from build123d import *

# Parameters (mm, degrees)
SKETCH_1_W                = 50
SKETCH_1_H                = 80
EXTRUDE_1_DEPTH           = 20
CUT_EXTRUDE_1_DEPTH       = 18
CUT_EXTRUDE_1_DEPTH_BACK  = 48
SKETCH_2_W                = 40
SKETCH_2_H                = 40
CUT_EXTRUDE_2_DEPTH       = 25
CUT_EXTRUDE_2_DEPTH_BACK  = 50
SKETCH_3_R                = 1.45
SKETCH_5_W                = 20
SKETCH_5_H                = 20
EXTRUDE_3_DEPTH           = 10
SKETCH_6_W                = 20
SKETCH_6_H                = 20
EXTRUDE_4_DEPTH           = 10
SKETCH_11_W               = 70
SKETCH_11_H               = 5
EXTRUDE_6_DEPTH           = 20
SKETCH_12_R               = 2.5
CUT_EXTRUDE_6_DEPTH       = 26
CHAMFER_1_SIZE            = 10
SKETCH_14_W               = 25
SKETCH_14_H               = 15
EXTRUDE_7_DEPTH           = 20
CHAMFER_2_SIZE            = 3
CHAMFER_3_SIZE            = 2
CUT_EXTRUDE_8_DEPTH       = 30
CUT_EXTRUDE_8_DEPTH_BACK  = 57
SKETCH_17_R               = 1.45
SKETCH_18_W               = 26.067158979
SKETCH_18_H               = 13.506639349
CUT_EXTRUDE_9_DEPTH       = 42
SKETCH_19_RX              = 28.99919082
SKETCH_19_RY              = 15.360713199
CUT_EXTRUDE_10_DEPTH      = 42
FILLET_1_R                = 7
EXTRUDE_START             = -12
SKETCH_20_R               = 2.5
SKETCH_20_R_2             = 1.75
EXTRUDE_8_DEPTH           = 3.5
SKETCH_21_W               = 20
SKETCH_21_H               = 0.5
CUT_EXTRUDE_11_DEPTH      = 31
SKETCH_22_W               = 50
SKETCH_22_H               = 2
CUT_EXTRUDE_12_DEPTH      = 31
CUT_EXTRUDE_14_DEPTH      = 14
CUT_EXTRUDE_14_DEPTH_BACK = 53
SKETCH_24_R               = 1.45
SKETCH_25_R               = 1.45
CUT_EXTRUDE_16_DEPTH      = 26
SKETCH_26_R               = 4
CUT_EXTRUDE_17_DEPTH      = 10


with BuildPart() as part:
    # 草图1 → 凸台-拉伸1 (new body)
    with BuildSketch(Plane.XY):
        Rectangle(SKETCH_1_W, SKETCH_1_H)
    extrude(amount=EXTRUDE_1_DEPTH)

    # 草图2 → 切除-拉伸1 (cut, two sides: drawn at the far end of the back side and taken through both)
    with BuildSketch(Plane.XY.offset(20).offset(-CUT_EXTRUDE_1_DEPTH_BACK)):
        with Locations((-25, 0)):
            Rectangle(SKETCH_2_W, SKETCH_2_H)
        with Locations((25, 0)):
            Rectangle(SKETCH_2_W, SKETCH_2_H)
    extrude(amount=CUT_EXTRUDE_1_DEPTH + CUT_EXTRUDE_1_DEPTH_BACK, mode=Mode.SUBTRACT)

    # 草图3 → 切除-拉伸2 (cut, two sides: drawn at the far end of the back side and taken through both)
    with BuildSketch(Plane.XY.offset(20).offset(-CUT_EXTRUDE_2_DEPTH_BACK)):
        with Locations(Location((9.925, -24.661145618, 0), (0, 0, 180))):
            Circle(SKETCH_3_R)
        with Locations(Location((19.775, -24.661145618, 0), (0, 0, 180))):
            Circle(SKETCH_3_R)
        with Locations(Location((9.925, 24.761145618, 0), (0, 0, 180))):
            Circle(SKETCH_3_R)
        with Locations(Location((19.775, 24.761145618, 0), (0, 0, 180))):
            Circle(SKETCH_3_R)
        with Locations(Location((-9.925, 24.761145618, 0), (0, 0, 180))):
            Circle(SKETCH_3_R)
        with Locations(Location((-19.775, 24.761145618, 0), (0, 0, 180))):
            Circle(SKETCH_3_R)
        with Locations(Location((-9.925, -24.661145618, 0), (0, 0, 180))):
            Circle(SKETCH_3_R)
        with Locations(Location((-19.775, -24.661145618, 0), (0, 0, 180))):
            Circle(SKETCH_3_R)
    extrude(amount=CUT_EXTRUDE_2_DEPTH + CUT_EXTRUDE_2_DEPTH_BACK, mode=Mode.SUBTRACT)

    # 草图5 → 凸台-拉伸3 (add)
    with BuildSketch(Plane(origin=(25, 0, 0), x_dir=(0, 0, -1), z_dir=(1, 0, 0))):
        with Locations((-10, -30)):
            Rectangle(SKETCH_5_W, SKETCH_5_H)
    extrude(amount=EXTRUDE_3_DEPTH)

    # 草图6 → 凸台-拉伸4 (add)
    with BuildSketch(Plane.ZY.offset(25)):
        with Locations((10, -30)):
            Rectangle(SKETCH_6_W, SKETCH_6_H)
    extrude(amount=EXTRUDE_4_DEPTH)

    # 草图11 → 凸台-拉伸6 (add)
    with BuildSketch(Plane.XY.offset(20)):
        with Locations((0, -42.5)):
            Rectangle(SKETCH_11_W, SKETCH_11_H)
    extrude(amount=-EXTRUDE_6_DEPTH)

    # 草图12 → 切除-拉伸6 (cut)
    with BuildSketch(Plane.XY.offset(20)):
        with Locations((27, -37)):
            Circle(SKETCH_12_R)
        with Locations(Location((-27, -37, 0), (0, 0, 180))):
            Circle(SKETCH_12_R)
    extrude(amount=-CUT_EXTRUDE_6_DEPTH, mode=Mode.SUBTRACT)

    # 倒角1
    chamfer_1_edges = [part.edges().sort_by_distance(p)[0] for p in [
        (35, -20, 10),
        (-35, -20, 10),
    ]]
    chamfer(chamfer_1_edges, length=CHAMFER_1_SIZE)

    # 草图14 → 凸台-拉伸7 (add)
    with BuildSketch(Plane.XY.offset(20)):
        with Locations((0, -45)):
            Rectangle(SKETCH_14_W, SKETCH_14_H)
    extrude(amount=-EXTRUDE_7_DEPTH)

    # 倒角2
    chamfer_2_edges = [part.edges().sort_by_distance(p)[0] for p in [
        (12.5, -52.5, 10),
        (-12.5, -52.5, 10),
    ]]
    chamfer(chamfer_2_edges, length=CHAMFER_2_SIZE)

    # 倒角3
    chamfer_3_edges = [part.edges().sort_by_distance(p)[0] for p in [
        (0, -52.5, 0),
        (0, -52.5, 20),
    ]]
    chamfer(chamfer_3_edges, length=CHAMFER_3_SIZE)

    # 草图17 → 切除-拉伸8 (cut, two sides: drawn at the far end of the back side and taken through both)
    with BuildSketch(Plane(origin=(0, 0, 0), x_dir=(-1, 0, 0), z_dir=(0, 0, -1)).offset(-CUT_EXTRUDE_8_DEPTH_BACK)):
        with Locations((15, 33)):
            Circle(SKETCH_17_R)
        with Locations((-15, 33)):
            Circle(SKETCH_17_R)
    extrude(amount=CUT_EXTRUDE_8_DEPTH + CUT_EXTRUDE_8_DEPTH_BACK, mode=Mode.SUBTRACT)

    # 草图18 → 切除-拉伸9 (cut)
    with BuildSketch(Plane.XY.offset(20)):
        with Locations((-0.53357949, -51.753319675)):
            Rectangle(SKETCH_18_W, SKETCH_18_H)
    extrude(amount=-CUT_EXTRUDE_9_DEPTH, mode=Mode.SUBTRACT)

    # 草图19 → 切除-拉伸10 (cut)
    with BuildSketch(Plane.XY.offset(20)):
        with Locations(Location((0, -56.905793797), (0, 0, 0))):
            Ellipse(SKETCH_19_RX, SKETCH_19_RY)
    extrude(amount=-CUT_EXTRUDE_10_DEPTH, mode=Mode.SUBTRACT)

    # 圆角1
    fillet_1_edges = [part.edges().sort_by_distance(p)[0] for p in [
        (-35, -45, 10),
        (35, -45, 10),
    ]]
    fillet(fillet_1_edges, radius=FILLET_1_R)

    # 草图20 → 凸台-拉伸8 (add)
    # profile 1 of 2: a face of its own
    with BuildSketch(Plane(origin=(0, 0, 0), x_dir=(-1, 0, 0), z_dir=(0, 0, -1)).offset(EXTRUDE_START)):
        with Locations((27, -37)):
            Circle(SKETCH_20_R)
        with Locations((27, -37)):
            Circle(SKETCH_20_R_2, mode=Mode.SUBTRACT)
    # profile 2 of 2: a face of its own
    with BuildSketch(Plane(origin=(0, 0, 0), x_dir=(-1, 0, 0), z_dir=(0, 0, -1)).offset(EXTRUDE_START)):
        with Locations(Location((-27, -37, 0), (0, 0, 180))):
            Circle(SKETCH_20_R)
        with Locations((-27, -37)):
            Circle(SKETCH_20_R_2, mode=Mode.SUBTRACT)
    extrude(amount=EXTRUDE_8_DEPTH)

    # 草图21 → 切除-拉伸11 (cut)
    with BuildSketch(Plane(origin=(0, 0, 0), x_dir=(-1, 0, 0), z_dir=(0, 0, -1))):
        with Locations((-15, 20.25)):
            Rectangle(SKETCH_21_W, SKETCH_21_H)
        with Locations((15, 20.25)):
            Rectangle(SKETCH_21_W, SKETCH_21_H)
    extrude(amount=-CUT_EXTRUDE_11_DEPTH, mode=Mode.SUBTRACT)

    # 草图22 → 切除-拉伸12 (cut)
    with BuildSketch(Plane(origin=(0, 0, 0), x_dir=(-1, 0, 0), z_dir=(0, 0, -1))):
        with Locations((0, 39)):
            Rectangle(SKETCH_22_W, SKETCH_22_H)
    extrude(amount=-CUT_EXTRUDE_12_DEPTH, mode=Mode.SUBTRACT)

    # 草图24 → 切除-拉伸14 (cut, two sides: drawn at the far end of the back side and taken through both)
    with BuildSketch(Plane(origin=(0, 0, 0), x_dir=(-1, 0, 0), z_dir=(0, 0, -1)).offset(-CUT_EXTRUDE_14_DEPTH_BACK)):
        with Locations((0, -33)):
            Circle(SKETCH_24_R)
    extrude(amount=CUT_EXTRUDE_14_DEPTH + CUT_EXTRUDE_14_DEPTH_BACK, mode=Mode.SUBTRACT)

    # 草图25 → 切除-拉伸16 (cut)
    with BuildSketch(Plane(origin=(0, 0, 0), x_dir=(-1, 0, 0), z_dir=(0, 0, -1))):
        with Locations((0, 22)):
            Circle(SKETCH_25_R)
    extrude(amount=-CUT_EXTRUDE_16_DEPTH, mode=Mode.SUBTRACT)

    # 草图26 → 切除-拉伸17 (cut)
    with BuildSketch(Plane(origin=(0, 38, 0), x_dir=(1, 0, 0), z_dir=(0, 1, 0))):
        with Locations(Location((0, -10, 0), (0, 0, 270))):
            Circle(SKETCH_26_R)
    extrude(amount=-CUT_EXTRUDE_17_DEPTH, mode=Mode.SUBTRACT)


solid = part.part
For this review, take the finished solid that the model builds, in its own axes (mm). A direction names the side the tool comes from. Give positions to 0.01 mm unless a question says otherwise; leave off trailing zeros. Loops run counter-clockwise (first coordinate to the right, second up) from the corner with the lowest first, then second, coordinate; pieces in that order, holes last. Notation, with made-up numbers: M 80.5,-23 L 123.5,-23 A10 cw 123.5,-12 Z; hole C -3.75,-27 d4. An arc over 180 degrees is marked long. Answer as a JSON object with one key per item and string values. Group by question number.
Q1. Insertion check: P1, Ø10, axis at x = -5, z = 15, coming from the -Y side; P2, Ø1.5, axis at x = 26, y = -36, coming from the -Z side; P3, Ø3, axis at x = -27, y = -37, coming from the +Z side; P4, Ø8, axis at x = -13, z = 7, coming from the -Y side. Each pin has a flat end and moves straight along its axis. Give the tip position at first contact, or say it passes through.
Q2. Tool access review of faces 5 (the cylindrical face through (25.16, -35.31, 16.06)), 6 (the flat face through (0, 28, 10)), 7 (the flat face through (15, 20.5, 10)), 8 (the cylindrical face through (25.16, -35.31, 4.31)), 9 (the flat face through (-25, 29, 10)): name each direction out of +Z, -Z, +X, -X, +Y, -Y from which nothing blocks a thin tool from reaching the whole face with its end or side.
Q3. Add section A-A on y = 33. Give the boundary of the cut face in (x, z).
Q4. Mouldability with a two-part tool opening along X and no side actions: class faces 1 (the flat face through (5, 0, 10)), 2 (the cylindrical face through (-26.46, -34.56, 16.06)), 3 (the flat face through (28, -39, 8.5)), 4 (the flat face through (0, -12, 0)) as +X half, -X half, draft (parallel to the pull), parting line (faces both ways), or undercut.
Q5. Add section C-C on x = -27. Give the boundary of the cut face in (y, z).
Q6. Add section B-B on y = 22. Give the boundary of the cut face in (x, z).
Q7. Add section D-D on y = -37. Give the boundary of the cut face in (x, z).
Q8. For probe 1 along X at (y, z) = (-37, 17.75); probe 2 along X at (y, z) = (36.25, 10); probe 3 along X at (y, z) = (-23.5, 16.5), list the stretches that pass through material, from the lowest coordinate up. Write a range as [from, to].
Checked values:
{
 "1": {"P1": "y = -42.49", "P2": "z = 8.5", "P3": "through", "P4": "y = -44.46"},
 "2": {"face 5": "+Z", "face 6": "+Y", "face 7": "+Z, -Z, +X", "face 8": "-Z", "face 9": "+Z, -Z, -X, +Y"},
 "3": {"outline": "M -25,0 L -16.45,0 L -16.45,20 L -25,20 Z; M -13.55,0 L 13.55,0 L 13.55,20 L -13.55,20 Z; M 16.45,0 L 25,0 L 25,20 L 16.45,20 Z; hole C 0,10 d8"},
 "4": {"face 1": "+X half", "face 2": "undercut", "face 3": "undercut", "face 4": "draft"},
 "5": {"outline": "M -45,0 L -39.5,0 L -39.5,8.5 L -38.75,8.5 L -38.75,12 L -39.5,12 L -39.5,20 L -45,20 Z; M -35.25,8.5 L -34.5,8.5 L -34.5,0 L -22,0 L -22,20 L -34.5,20 L -34.5,12 L -35.25,12 Z"},
 "6": {"outline": "M -25,0 L -1.45,0 L -1.45,20 L -25,20 Z; M 1.45,0 L 25,0 L 25,20 L 1.45,20 Z"},
 "7": {"outline": "M -35,0 L -29.5,0 L -29.5,8.5 L -28.75,8.5 L -28.75,12 L -29.5,12 L -29.5,20 L -35,20 Z; M -25.25,8.5 L -24.5,8.5 L -24.5,0 L 24.5,0 L 24.5,8.5 L 25.25,8.5 L 25.25,12 L 24.5,12 L 24.5,20 L -24.5,20 L -24.5,12 L -25.25,12 Z; M 28.75,8.5 L 29.5,8.5 L 29.5,0 L 35,0 L 35,20 L 29.5,20 L 29.5,12 L 28.75,12 Z"},
 "8": {"probe 1": "[-35, -29.5], [-24.5, 24.5], [29.5, 35]", "probe 2": "[-25, -4], [4, 25]", "probe 3": "[-28.5, -20.64], [-18.91, -10.79], [-9.06, 9.06], [10.79, 18.91], [20.64, 28.5]"}
}
